Check sheet for the modelled part. Datum: model origin and axes. Units: mm. A direction names the side the tool comes from. Give positions to 0.01 mm unless a question says otherwise; leave off trailing zeros. Write each loop counter-clockwise with the first axis right and the second up, starting at its lowest first coordinate (ties: lowest second). Pieces come first, ordered by that corner, then holes. Notation, with made-up numbers: M -20.75,86.25 L -16.75,86.25 A22 cw -16.75,110.25 Z; hole C 2.25,46.5 d10. An arc over 180 degrees is marked long. Write item = value, one per line. Start each with the question number.
1) Set-up check for faces 4 (the face through (57.85, -4.17, 5.45)), 5 (the face through (-51, 32, 1)), 6 (the face through (-72.23, -87.63, 2.34)): record each of +Z, -Z, +X, -X, +Y, -Y from which the full face is reachable in a straight line by a thin tool's end or side.
2) Sectioned sample at A-A, the plane x = -7.5. Record the cut outline in (y, z), then the cut area to 3 significant figures.
3) Sectioned sample at C-C, the plane y = 78. Record the cut outline in (x, z).
4) Scan lines: L1, parallel to Y at x = -36, z = 2.75; L2, parallel to Z at x = 58, y = 24; L3, parallel to Y at x = -42, z = 3.5. Record each from-to range of solid material in increasing order.
5) Sectioned sample at D-D, the plane y = -60.5. Record the cut outline in (x, z).
6) Draft check along X on faces 1 (the face through (-73.5, 53, 5)), 2 (the face through (-51, 8.797, 5)), 3 (the face through (25, 73, 1)). Enter one of: pulls with the +X half, pulls with the -X half, needs draft (parallel to the pull), parting line crosses it, or undercut.
7) Gauge pin test, flat ends, axial feed: pin 1 (1.8 mm diameter, centred on x = -50.5, y = 71.5, fed in from +Z); pin 2 (5 mm diameter, centred on x = 25.5, y = 73, fed in from +Z); pin 3 (5 mm diameter, centred on y = 18, z = 3.5, fed in from +X). Record the tip position at first contact, or that the pin passes through.
from build123d import *

# Parameters (mm, degrees)
SKETCH_1_W          = 147
SKETCH_1_H          = 194
EXTRUDE_1_DEPTH     = 2
CUT_EXTRUDE_1_DEPTH = 122.717911582
EXTRUDE_2_DEPTH     = 7
EXTRUDE_12_DEPTH    = 2
EXTRUDE_13_DEPTH    = 7
SKETCH_9_W          = 30
SKETCH_9_H          = 7
CUT_EXTRUDE_2_DEPTH = 8
CUT_EXTRUDE_3_DEPTH = 165.668883446
CUT_EXTRUDE_4_DEPTH = 125.640523105
FILLET_1_R          = 10
SKETCH_15_R         = 3
CUT_EXTRUDE_5_DEPTH = 1


with BuildPart() as part:
    # 草图1 → 凸台-拉伸1 (new body)
    with BuildSketch(Plane.XY):
        Rectangle(SKETCH_1_W, SKETCH_1_H)
    extrude(amount=EXTRUDE_1_DEPTH)

    # 草图3 → 切除-拉伸1 (cut, through all)
    with BuildSketch(Plane.XY.offset(2)):
        Polygon((53.23522436, -12.067612089), (54.895536272, -9.227626556), (56.571241133, -6.361232674), (59.922644339, -0.628613065), (61.598241137, 2.237687122), (63.273937257, 5.103974498), (64.949644621, 7.97037266), (66.685320016, 10.939281948), (68.474937854, 14.800520519), (69.965464928, 18.751847603), (71.186607188, 22.785544771), (72.160677785, 26.878843337), (72.909711272, 31.009687619), (73.455390422, 35.156598129), (73.81891313, 39.298369912), (74.02249192, 43.433108573), (74.02249192, 45), (75.723074591, 45), (75.723074591, -104.819726649), (48.204220565, -104.819726649), align=None)
    extrude(amount=-CUT_EXTRUDE_1_DEPTH, mode=Mode.SUBTRACT)

    # 草图4 → 凸台-拉伸2 (add)
    with BuildSketch(Plane.XY.offset(2)):
        with BuildLine():
            Line((-26.359304292, 7.671510526), (-26.359304292, -2.050234399))
            Line((-26.359304292, -2.050234399), (-26.291229671, -2.727324911))
            Line((-26.291229671, -2.727324911), (-26.056539241, -3.484651495))
            Line((-26.056539241, -3.484651495), (-25.685607127, -4.168114429))
            Line((-25.685607127, -4.168114429), (-25.196433295, -4.761489945))
            Line((-25.196433295, -4.761489945), (-24.602579713, -5.251299759))
            Line((-24.602579713, -5.251299759), (-23.918848604, -5.622103659))
            Line((-23.918848604, -5.622103659), (-23.16220103, -5.856620758))
            Line((-23.16220103, -5.856620758), (-22.484966559, -5.924875416))
            Line((-22.484966559, -5.924875416), (33.258451472, -5.924875416))
            ThreePointArc((33.258451472, -5.924875416), (35.166456954, -6.084261893), (37.021573693, -6.558003228))
            Line((37.021573693, -6.558003228), (38.696489946, -7.527643824))
            Line((38.696489946, -7.527643824), (40.372194808, -8.497858613))
            Line((40.372194808, -8.497858613), (43.723589271, -10.43804405))
            Line((43.723589271, -10.43804405), (45.399266369, -11.408242764))
            Line((45.399266369, -11.408242764), (47.074877038, -12.378342789))
            Line((47.074877038, -12.378342789), (48.808729273, -13.382197265))
            Line((48.808729273, -13.382197265), (49.23970493, -13.601689934))
            Line((49.23970493, -13.601689934), (53.032447862, -15.806020922))
            Line((53.032447862, -15.806020922), (48.628373423, -97))
            Line((48.628373423, -97), (-73.5, -97))
            Line((-73.5, -97), (-73.5, 8.797108615))
            Line((-73.5, 8.797108615), (-69.625285972, 8.797108615))
            Line((-69.625285972, 8.797108615), (-27.484917142, 8.797108615))
            Line((-27.484917142, 8.797108615), (-26.359304292, 7.671510526))
        make_face()
    extrude(amount=EXTRUDE_2_DEPTH)

    # 草图6 → 凸台-拉伸12 (add)
    with BuildSketch(Plane(origin=(0, 0, 0), x_dir=(-1, 0, 0), z_dir=(0, 0, -1))):
        Polygon((-61.598241137, 2.237687122), (-53.998328187, -10.762312878), (-55.206947225, -11.468882068), (-62.806860175, 1.531117932), align=None)
        Polygon((-73.5, 97), (73.5, 97), (73.5, -97), (74.9, -97), (74.9, 87), (74.9, 99.5), (-73.5, 99.5), align=None)
    extrude(amount=-EXTRUDE_12_DEPTH)

    # 草图7 → 凸台-拉伸13 (add)
    with BuildSketch(Plane.XY.offset(2)):
        Polygon((-74.9, 99.5), (-74.9, -97), (-73.5, -97), (-73.5, 98.5), (73.5, 98.5), (73.5, 99.5), align=None)
        Polygon((61.598241137, 2.237687122), (53.998328187, -10.762312878), (55.206947225, -11.468882068), (62.806860175, 1.531117932), align=None)
    extrude(amount=EXTRUDE_13_DEPTH)

    # 草图9 → 切除-拉伸2 (cut)
    with BuildSketch(Plane(origin=(0, 99.5, 0), x_dir=(1, 0, 0), z_dir=(0, 1, 0))):
        with Locations((58.5, -5.5)):
            Rectangle(SKETCH_9_W, SKETCH_9_H)
    extrude(amount=-CUT_EXTRUDE_2_DEPTH, mode=Mode.SUBTRACT)

    # 草图10 → 切除-拉伸3 (cut, through all)
    with BuildSketch(Plane(origin=(53.731702858, -2.914482352, 0), x_dir=(0, 0, -1), z_dir=(0.9985321738095838, -0.054161774962672445, 0))):
        Polygon((-9, -30.223821841), (-4, -94.223821841), (-4, -111.514790755), (-9, -111.514790755), (-9, -94.223821841), align=None)
    extrude(amount=-CUT_EXTRUDE_3_DEPTH, mode=Mode.SUBTRACT)

    # 草图11 → 切除-拉伸4 (cut, through all)
    with BuildSketch(Plane.XY.offset(4)):
        Polygon((-74.9, -90.299649087), (-74.9, -97), (48.628373423, -97), align=None)
    extrude(amount=-CUT_EXTRUDE_4_DEPTH, mode=Mode.SUBTRACT)

    # 圆角1
    fillet_1_edges = [part.edges().sort_by_distance(p)[0] for p in [
        (-74.9, -90.299649087, 2),
        (48.628373423, -97, 2),
    ]]
    fillet(fillet_1_edges, radius=FILLET_1_R)

    # 草图15 → 切除-拉伸5 (cut)
    with BuildSketch(Plane.XY.offset(2)):
        with Locations((-51.34000037, 70.5)):
            Circle(SKETCH_15_R)
        with Locations((-51.34000037, 32.300001397)):
            Circle(SKETCH_15_R)
        with Locations((24.859996084, 72.7)):
            Circle(SKETCH_15_R)
        with Locations((24.859996084, 34.700002149)):
            Circle(SKETCH_15_R)
        with Locations((49.459993167, 17.5)):
            Circle(SKETCH_15_R)
    extrude(amount=-CUT_EXTRUDE_5_DEPTH, mode=Mode.SUBTRACT)


solid = part.part
Data:
q1.face_4 = +Z, +Y
q1.face_5 = +Z
q1.face_6 = +Z, -Z, -X, -Y
q2.outline = M -93.96,0 L 99.5,0 L 99.5,9 L 98.5,9 L 98.5,2 L -5.92,2 L -5.92,9 L -29.86,9 L -93.96,4 Z
q2.area = 850 mm2
q3.outline = M -74.9,0 L 73.5,0 L 73.5,2 L -73.5,2 L -73.5,9 L -74.9,9 Z
q4.L1 = -92.41 to 8.8, 98.5 to 99.5
q4.L2 = 0 to 2
q4.L3 = -92.08 to 8.8, 98.5 to 99.5
q5.outline = M -74.9,0 L 50.61,0 L 50.61,6.86 L -74.9,6.32 Z
q6.face_1 = pulls with the +X half
q6.face_2 = needs draft
q6.face_3 = undercut
q7.pin_1 = 1
q7.pin_2 = 2
q7.pin_3 = 70.34
